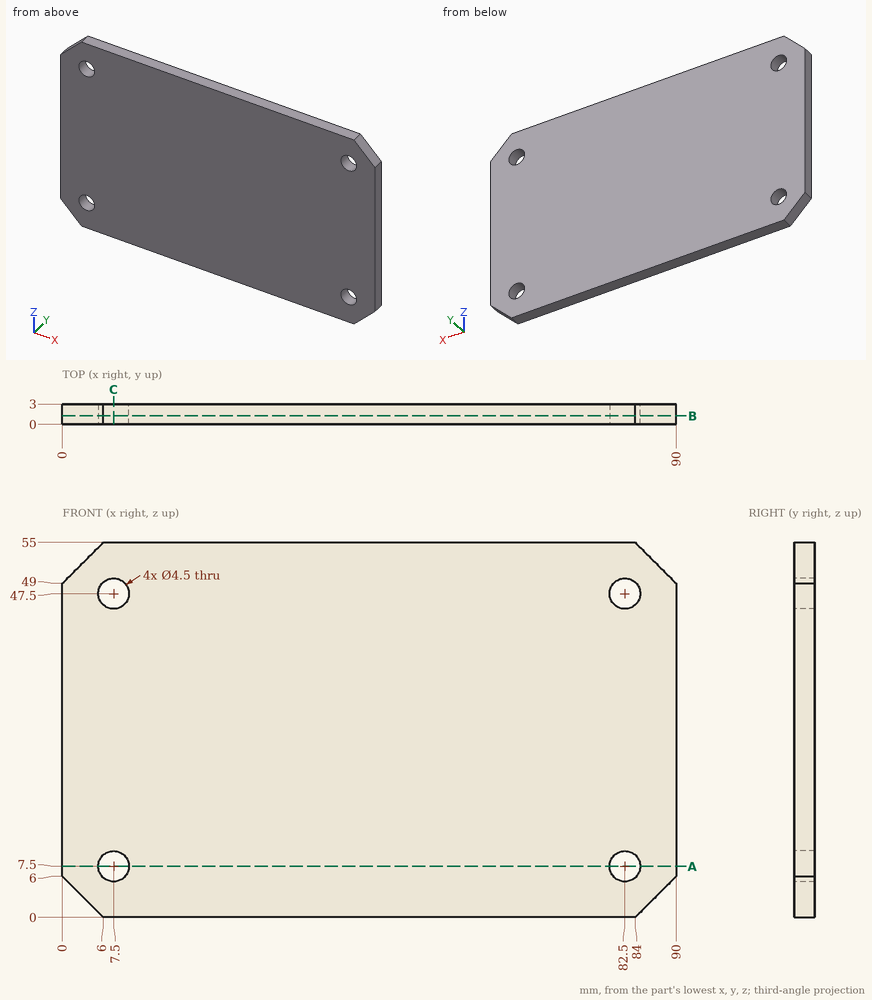
Design review of the part shown in the three views and the two pictorial views. Dimensions are in mm from the part's minimum x, y and z. Coordinates: 2 decimals unless noted, no trailing zeros. Order: outer loops, then holes, each group sorted by start corner. A loop starts at its lowest first (then second) coordinate and runs counter-clockwise, first axis right, second up.
1) Take a section at B-B, the plane y = 1.25. Give the boundary of the cut face in (x, z), and give its area (3 significant figures).
2) Wall thickness on line 1 along X through (y, z) = (0.7, 47.5); line 2 along Z through (x, y) = (82.5, 2); line 3 along X through (y, z) = (2.5, 6): over which ranges is each line inside the solid? List them lowest first.
3) Take a section at A-A, the plane z = 7.5. Give the boundary of the cut face in (x, y).
4) Take a section at C-C, the plane x = 7.5. Give the boundary of the cut face in (y, z), and give its area (3 significant figures).
Returned:
1. outline: (0, 6) - (6, 0) - (84, 0) - (90, 6) - (90, 49) - (84, 55) - (6, 55) - (0, 49) - close; hole circle Ø4.5 at (7.5, 7.5); hole circle Ø4.5 at (7.5, 47.5); hole circle Ø4.5 at (82.5, 7.5); hole circle Ø4.5 at (82.5, 47.5)
1. area: 4,810 mm2
2. line 1: x = 0 to 5.25, 9.75 to 80.25, 84.75 to 90
2. line 2: z = 0 to 5.25, 9.75 to 45.25, 49.75 to 55
2. line 3: x = 0 to 5.82, 9.18 to 80.82, 84.18 to 90
3. outline: (0, 0) - (5.25, 0) - (5.25, 3) - (0, 3) - close; (9.75, 0) - (80.25, 0) - (80.25, 3) - (9.75, 3) - close; (84.75, 0) - (90, 0) - (90, 3) - (84.75, 3) - close
4. outline: (0, 0) - (3, 0) - (3, 5.25) - (0, 5.25) - close; (0, 9.75) - (3, 9.75) - (3, 45.25) - (0, 45.25) - close; (0, 49.75) - (3, 49.75) - (3, 55) - (0, 55) - close
4. area: 138 mm2
